from build123d import *

# Parameters (mm, degrees)
F0_W      = 4
F0_H      = 4
F1_DEPTH  = 0.8
F4_DEPTH  = 1.5
F5_R      = 1
F6_DEPTH  = 10.2624610432
F7_R      = 1.49999
F8_R      = 0.49999
F10_DEPTH = 1


# Not quite as in the source:
# - a fillet or chamfer is up to 0.001 mm smaller than in the source, because OpenCascade refuses the exact size


with BuildPart() as f1:
    # F0 (on Top) → F1 (new body)
    with BuildSketch(Plane.XY):
        with Locations((3, 2)):
            Rectangle(F0_W, F0_H)
    extrude(amount=F1_DEPTH)

    # F3 (on offset) → F4 (join, symmetric)
    with BuildSketch(Plane.YZ.offset(2.5)):
        Polygon((0.5, 0.8), (3.5, 0.8), (10.2614610432, 15.3), (10.2614610432, 19.8), (7.2614610432, 19.8), (7.2614610432, 15.3), align=None)
    extrude(amount=F4_DEPTH, both=True)

    # F5 (on face) → F6 (cut, through all)
    with BuildSketch(Plane(origin=(0, 10.2614610432, 0), x_dir=(-1, 0, 0), z_dir=(0, 1, 0))):
        with Locations((-2.5, 17.8)):
            Circle(F5_R)
    extrude(amount=-F6_DEPTH, mode=Mode.SUBTRACT)

    # F7 (radius 1.5 in the source; OpenCascade refuses exactly that, so slightly less here)
    f7_edges = [f1.edges().sort_by_distance(p)[0] for p in [
        (1, 8.761461, 19.8),
        (4, 8.761461, 19.8),
    ]]
    fillet(f7_edges, radius=F7_R)

    # F8 (radius 0.5 in the source; OpenCascade refuses exactly that, so slightly less here)
    f8_edges = [f1.edges().sort_by_distance(p)[0] for p in [
        (1, 6.880731, 8.05),
        (1, 10.261461, 16.800005),
        (3.560663, 10.261461, 19.360663),
        (4, 6.880731, 8.05),
        (1, 3.880731, 8.05),
        (1, 7.261461, 16.800005),
        (4, 3.880731, 8.05),
    ]]
    fillet(f8_edges, radius=F8_R)

    # F9 (on face) → F10 (join)
    with BuildSketch(Plane.YZ.offset(5)):
        with BuildLine():
            Line((0, 2.3), (0, 0.8))
            Line((0, 0.8), (4, 0.8))
            Line((4, 0.8), (4, 2.3))
            ThreePointArc((4, 2.3), (2, 4.3), (0, 2.3))
        make_face()
    extrude(amount=-F10_DEPTH)


solid = f1.part
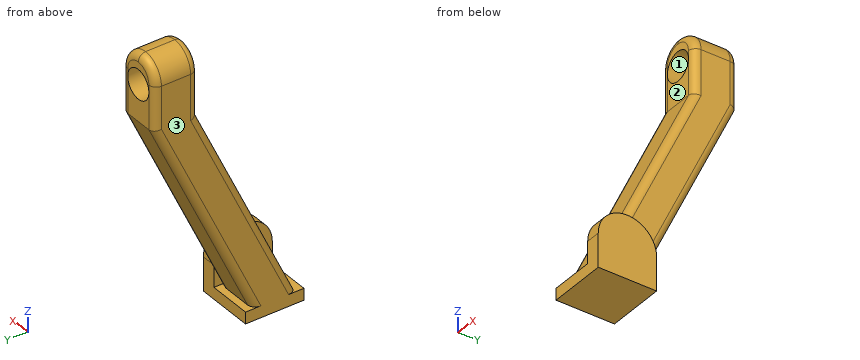
The listing builds one solid part. Answer for the finished solid, in the listing's coordinates (mm). Face numbers are marked on the shaded views. Give positions to 0.01 mm unless a question says otherwise; leave off trailing zeros. Use one line per item in the form item = value.
1) Consider probe 1 along Z at (x, y) = (2.5, 8.3); probe 2 along Z at (x, y) = (2.5, 9.05); probe 3 along Y at (x, z) = (3.1, 16.75). Determine where each line is inside the solid, lowest interval first. Write a range as [from, to].
Verdict:
probe_1 = [11.09, 16.8], [18.8, 19.8]
probe_2 = [12.7, 16.8], [18.8, 19.8]
probe_3 = [7.26, 10.26]
2) Each of these flat-tipped pins is pushed along its axis until it touches: pin 1 (2 mm diameter, centred on y = 6.5, z = 10.5, fed in from +X); pin 2 (1.6 mm diameter, centred on x = 2.5, z = 17, fed in from -Y); pin 3 (1.2 mm diameter, centred on x = 2.5, z = 17.8, fed in from +Y); pin 4 (0.5 mm diameter, centred on x = 2.5, y = 0.5, fed in from +Z). Where does it stop, or does it pass through?
Verdict:
pin_1 = 4
pin_2 = 7.26
pin_3 = through
pin_4 = 1.34
3) The mould has two halves that part along X. Classify the marked faces 1, 2 and 3: released by +X, released by -X, zero draft, split by the parting line, or undercut.
Verdict:
face_1 = undercut
face_2 = zero draft
face_3 = released by -X
